Build history of the part. All positions in model axes, mm. A direction names the side the tool comes from. Round coordinates to 2 decimals unless told otherwise and drop trailing zeros. Order: outer loops, then holes, each group sorted by start corner. A loop starts at its lowest first (then second) coordinate and runs counter-clockwise, first axis right, second up. Notation, with made-up numbers: M 39,19 L 91,19 A34 cw 91,55 Z; hole C -28.5,33.25 d3. An arc over 180 degrees is marked long. One line per item, written item: value. Start each with the question number.
Item 1: Band-saw the part on A-A, the plane z = -52. Write the cut outline in (x, y), then the cut area to 3 significant figures.
Item 2: Band-saw the part on B-B, the plane y = -15. Give the number of separate pieces and of enclosed holes in the cut face, then the cut area to 3 significant figures.
Item 3: Tool access for faces 4 (the flat face through (9.048, -15, -63)), 5 (the cylindrical face through (32.76, -1.83, -35.48)), 6 (the flat face through (28, -29.1, -24)), 7 (the flat face through (18.448, -9, -63)), 8 (the flat face through (54.748, -15, -33)): list every direction of +Z, -Z, +X, -X, +Y, -Y with a clear straight run to the whole face (end or side of a thin tool).
Item 4: Pin check, flat tips, straight feed: pin 1 (6 mm diameter, centred on y = -11.5, z = -27.5, fed in from -X); pin 2 (5 mm diameter, centred on y = -9.5, z = -15, fed in from +X); pin 3 (4 mm diameter, centred on x = 28, z = -24.5, fed in from -Y); pin 4 (5 mm diameter, centred on x = 56, z = -57.5, fed in from +Y). Stop position of each tip, or through.
Item 5: Probe L1, parallel to X at y = -15, z = -1.25; L2, parallel to X at y = -6.75, z = -26.5; L3, parallel to X at y = -7, z = -55. List the from-to ranges inside material, lowest first.
Item 6: Band-saw the part on C-C, the plane x = 68. Write the cut outline in (y, z), then the cut area to 3 significant figures.
Item 7: Band-saw the part on D-D, the plane y = -3. Write the cut outline in (x, z).
Item 8: Two-plate mould, pull along Y, no slides. Class faces 1 (the cylindrical face through (11.3, -0.4, -1.4)), 2 (the cylindrical face through (9.532, -28.168, -30.408)), 3 (the cylindrical face through (4.33, -13.4, -1.86)): +Y half, -Y half, draft (parallel to the pull), parting line (faces both ways), or undercut.
Autodesk Inventor part; units mm, degrees
ref_plane "YZ Plane" through (0, 0, 0) normal (1, 0, 0) x (0, 1, 0)
ref_plane "XZ Plane" through (0, 0, 0) normal (0, 1, 0) x (-1, 0, 0)
ref_plane "XY Plane" through (0, 0, 0) normal (0, 0, 1) x (1, 0, 0)
sketch "Skizze1" plane through (0, 0, 0) normal (0, 0, 1) x (1, 0, 0)
  line L0 (13.15, 0) -> (71.15, 0)
  line L1 (71.15, -30) -> (13.15, -30)
  arc A0 (1.7779, -11.1719) -> (1.7779, -18.8281) centre (6.398, -15) ccw
  arc A1 (82.5191, -18.827) -> (82.5191, -11.173) centre (77.898, -15) ccw
  line L2 (13.15, 0) -> (71.15, 0)
  line L3 (71.15, -30) -> (13.15, -30)
  arc A2 (13.15, 0) -> (9.6849, -1.6289) centre (13.15, -4.5) ccw
  arc A3 (9.6849, -28.3711) -> (13.15, -30) centre (13.15, -25.5) ccw
  arc A4 (71.15, -30) -> (74.6158, -28.3702) centre (71.15, -25.5) ccw
  arc A5 (74.6158, -1.6298) -> (71.15, 0) centre (71.15, -4.5) ccw
  line L4 (9.6849, -1.6289) -> (1.7779, -11.1719)
  line L5 (1.7779, -18.8281) -> (9.6849, -28.3711)
  line L6 (74.6158, -28.3702) -> (82.5191, -18.827)
  line L7 (74.6158, -1.6298) -> (82.5191, -11.173)
  line L8 (6.398, -15) -> (77.898, -15) construction
  point P0 (0, 0)
  point P1 (74.85, -30)
  dimension "d2" = 12
  dimension "d3" = 12
  dimension "d6" = 4.5
  dimension "d47" = 71.5
  dimension "d48" = 21
  dimension "d49" = 21
  dimension "d50" = 58
  dimension "d51" = 58
  dimension "d52" = 15
  dimension "d53" = 15
  dimension "d54" = 50.37
  dimension "d55" = 50.37
  dimension "d56" = 50.356
  dimension "d57" = 50.356
extrude "Extrusion1" add sketch "Skizze1" against normal blind 2.8
sketch "Skizze2" plane through (0, 0, 0) normal (0, 0, 1) x (1, 0, 0)
  arc A0 (1.7779, -11.1719) -> (1.7779, -18.8281) centre (6.398, -15) ccw
  point P0 (0, 0)
  point P1 (4.398, -15)
  point P2 (79.898, -15)
  dimension "d9" = 75.5
  dimension "d10" = 2
hole "Bohrung1" at (4.398, -15, 0) at (79.898, -15, 0) direction (0, 0, -1) diameter 3.2 end through all countersink diameter 5 countersink angle 90
sketch "Skizze3" plane through (0, 0, -2.8) normal (0, 0, -1) x (-1, 0, 0)
  circle A0 centre (-79.898, -15) radius 1.6
  arc A1 (-13.15, -30) -> (-9.6849, -28.3711) centre (-13.15, -25.5) ccw
  line L0 (-16.4119, -28.6) -> (-15.1466, -28.6)
  line L1 (-15.1466, -1.4) -> (-29.2653, -1.4)
  line L2 (-72.548, -29.1) -> (-11.748, -29.1)
  line L3 (-8.648, -26) -> (-8.648, -4)
  line L4 (-11.748, -0.9) -> (-72.548, -0.9)
  line L5 (-75.648, -4) -> (-75.648, -26)
  arc A2 (-75.648, -26) -> (-72.548, -29.1) centre (-72.548, -26) ccw
  arc A3 (-72.548, -0.9) -> (-75.648, -4) centre (-72.548, -4) ccw
  arc A4 (-8.648, -4) -> (-11.748, -0.9) centre (-11.748, -4) ccw
  arc A5 (-11.748, -29.1) -> (-8.648, -26) centre (-11.748, -26) ccw
  line L6 (-13.15, -30) -> (-71.15, -30)
  line L7 (-71.15, 0) -> (-13.15, 0)
  point P0 (0, 0)
  point P1 (-8.648, -0.9)
  point P2 (-75.648, -0.9)
  dimension "d20" = 67
  dimension "d21" = 4.25
  dimension "d22" = 3.1
  dimension "d44" = 28.2
  dimension "d45" = 0.9
  dimension "d46" = 0.9
extrude "Extrusion2" add sketch "Skizze3" along normal blind 10 contours A2 L5 A3 L4 A4 L3 A5 L2
sketch "Skizze4" plane through (0, 0, -12.8) normal (0, 0, -1) x (-1, 0, 0)
  line L0 (-11.748, -29.1) -> (-72.548, -29.1)
  line L1 (-8.648, -4) -> (-8.648, -26)
  line L2 (-11.748, -0.9) -> (-30.548, -0.9)
  line L3 (-33.648, -4) -> (-33.648, -26)
  line L4 (-30.548, -29.1) -> (-11.748, -29.1)
  line L5 (-8.648, -26) -> (-8.648, -4)
  arc A0 (-11.748, -29.1) -> (-8.648, -26) centre (-11.748, -26) ccw
  arc A1 (-8.648, -4) -> (-11.748, -0.9) centre (-11.748, -4) ccw
  arc A2 (-30.548, -0.9) -> (-33.648, -4) centre (-30.548, -4) ccw
  arc A3 (-33.648, -26) -> (-30.548, -29.1) centre (-30.548, -26) ccw
  point P0 (0, 0)
  point P1 (-33.648, -29.1)
  dimension "d25" = 25
  dimension "d26" = 3.1
  dimension "d27" = 0
  dimension "d28" = 3.1
extrude "Extrusion3" add sketch "Skizze4" along normal blind 46
sketch "Skizze5" plane through (0, 0, -58.8) normal (0, 0, -1) x (-1, 0, 0)
  line L0 (-8.648, -4) -> (-8.648, -26)
  line L1 (-11.748, -29.1) -> (-30.548, -29.1)
  line L2 (-9.848, -17.5) -> (-9.048, -17.5)
  line L3 (-9.048, -17.5) -> (-9.048, -12.7)
  line L4 (-9.048, -12.7) -> (-9.848, -12.7)
  line L5 (-9.848, -12.7) -> (-9.848, -17.5)
  line L6 (-30.548, -0.9) -> (-11.748, -0.9)
  line L7 (-18.448, -6.9) -> (-17.648, -6.9)
  line L8 (-17.648, -6.9) -> (-17.648, -11.7)
  line L9 (-17.648, -11.7) -> (-18.448, -11.7)
  line L10 (-18.448, -11.7) -> (-18.448, -6.9)
  line L11 (-18.448, -18.3) -> (-17.648, -18.3)
  line L12 (-17.648, -18.3) -> (-17.648, -23.1)
  line L13 (-17.648, -23.1) -> (-18.448, -23.1)
  line L14 (-18.448, -23.1) -> (-18.448, -18.3)
  point P0 (0, 0)
  dimension "d31" = 0.4
  dimension "d33" = 0.8
  dimension "d35" = 4.8
  dimension "d37" = 11.6
  dimension "d62" = 0.8
  dimension "d63" = 0.8
  dimension "d64" = 4.8
  dimension "d65" = 4.8
  dimension "d66" = 6
  dimension "d67" = 6
  dimension "d68" = 0
  dimension "d69" = 9
extrude "Extrusion4" add sketch "Skizze5" along normal blind 8
sketch "Skizze6" plane through (0, 0, -12.8) normal (0, 0, -1) x (-1, 0, 0)
  line L0 (-30.548, -29.1) -> (-72.548, -29.1)
  line L1 (-71.648, -1.8) -> (-57.848, -1.8)
  line L2 (-54.748, -4.9) -> (-54.748, -25.1)
  line L3 (-74.748, -25.1) -> (-74.748, -4.9)
  arc A0 (-71.648, -1.8) -> (-74.748, -4.9) centre (-71.648, -4.9) ccw
  arc A1 (-54.748, -4.9) -> (-57.848, -1.8) centre (-57.848, -4.9) ccw
  arc A2 (-57.848, -28.2) -> (-54.748, -25.1) centre (-57.848, -25.1) ccw
  arc A3 (-74.748, -25.1) -> (-71.648, -28.2) centre (-71.648, -25.1) ccw
  line L4 (-72.548, -0.9) -> (-30.548, -0.9)
  line L5 (-75.648, -26) -> (-75.648, -4)
  line L6 (-33.648, -26) -> (-33.648, -4)
  line L7 (-71.648, -28.2) -> (-57.848, -28.2)
  point P0 (0, 0)
  point P1 (-54.748, -29.1)
  dimension "d40" = 20
  dimension "d41" = 3.1
  dimension "d58" = 0.9
  dimension "d59" = 0.9
  dimension "d60" = 0.9
  dimension "d61" = 26.4
extrude "Extrusion5" add sketch "Skizze6" along normal blind 40.2
equation "\"d2\" = d3"
properties part number "Schurter_CDG4_4101_151"
Output:
1. outline: M 8.65,-26 A3.1 ccw 11.75,-29.1 L 30.55,-29.1 A3.1 ccw 33.65,-26 L 33.65,-4 A3.1 ccw 30.55,-0.9 L 11.75,-0.9 A3.1 ccw 8.65,-4 Z; M 54.75,-25.1 A3.1 ccw 57.85,-28.2 L 71.65,-28.2 A3.1 ccw 74.75,-25.1 L 74.75,-4.9 A3.1 ccw 71.65,-1.8 L 57.85,-1.8 A3.1 ccw 54.75,-4.9 Z
1. area: 1,220 mm²
2. separate pieces: 3
2. enclosed holes: 0
2. area: 2,840 mm²
3. face 4: -Z, -X, +Y, -Y
3. face 5: -Z, +Y
3. face 6: -Z, +X, -X, -Y
3. face 7: -Z, +X, +Y, -Y
3. face 8: -Z, +Y, -Y
4. pin 1: stops at x = 8.65
4. pin 2: stops at x = 75.65
4. pin 3: stops at y = -29.1
4. pin 4: passes through
5. L1: x = 0.4 to 2.8, 6 to 78.3, 81.5 to 83.9
5. L2: x = 8.65 to 33.65, 54.75 to 74.75
5. L3: x = 8.65 to 33.65
6. outline: M -30,-2.8 L -29.1,-2.8 L -29.1,-12.8 L -28.2,-12.8 L -28.2,-53 L -1.8,-53 L -1.8,-12.8 L -0.9,-12.8 L -0.9,-2.8 L 0,-2.8 L 0,0 L -30,0 Z
6. area: 1,430 mm²
7. outline: M 8.55,-2.8 L 8.81,-2.8 L 8.81,-58.8 L 33.48,-58.8 L 33.48,-12.8 L 55.4,-12.8 L 55.4,-53 L 74.1,-53 L 74.1,-12.8 L 75.48,-12.8 L 75.48,-2.8 L 75.75,-2.8 L 75.75,0 L 8.55,0 Z
8. face 1: +Y half
8. face 2: -Y half
8. face 3: undercut
